Here's how the part is built. I have some questions about the finished solid (model axes, mm). A direction names the side the tool comes from. Coordinates: 2 decimals unless noted, no trailing zeros. Write each loop counter-clockwise with the first axis right and the second up, starting at its lowest first coordinate (ties: lowest second). Pieces come first, ordered by that corner, then holes.
Item 1: Please list where these lines run through material, in increasing order: line 1 (Z direction, x = 13, y = 0); line 2 (Y direction, x = 5.5, z = 0); line 3 (X direction, y = 2.25, z = 13.5).
Item 2: I want a section at C-C (x = 12.5). Please give me the cut outline in (y, z).
Item 3: I'm going to push flat-ended pins straight in: P1, Ø2.5, axis at y = -0.5, z = -12, coming from the +X side; P2, Ø5, axis at x = 5, y = -3.5, coming from the -Z side; P3, Ø1.8, axis at x = 7.5, y = 5, coming from the -Z side; P4, Ø1.5, axis at y = 1, z = 13, coming from the -X side. Where does each tip first touch, or does it pass through?
Item 4: If we mould it in two halves opening along Z, with no side actions, what happens to faces 4 (the face through (8, 6.78, 0)), 5 (the face through (0, 0.1, -5.5)), 6 (the face through (8, 6, 2)), 7 (the face through (14, 0, 15))? For each: pulls with the +Z half, pulls with the -Z half, needs draft (parallel to the pull), parting line crosses it, or undercut.
Item 5: I want a section at A-A (y = 0). Please give me the cut outline in (x, z), and give its area (3 significant figures).
Item 6: I want a section at D-D (x = 7.75). Please give me the cut outline in (y, z), and give its area (3 significant figures).
Item 7: I want a section at B-B (z = 0). Please give me the cut outline in (x, y).
Item 8: For faces 1 (the face through (14, 2.5, 12)), 2 (the face through (2, -2.5, -12)), 3 (the face through (14, -2.5, 12)), which set-ups out of +Z, -Z, +X, -X, +Y, -Y let a thin tool reach every point of the face, with its end or its side?
from build123d import *

# Parameters (mm, degrees)
SKETCH1_R           = 9
BOSS_EXTRUDE1_DEPTH = 17
SKETCH3_W           = 5
SKETCH3_H           = 15
BOSS_EXTRUDE3_DEPTH = 2.5
SKETCH4_R           = 5
CUT_EXTRUDE1_DEPTH  = 25.392621835


with BuildPart() as part:
    # Sketch1 → Boss-Extrude1 (new body)
    with BuildSketch(Plane(origin=(0, 0, 0), x_dir=(0, 0, -1), z_dir=(1, 0, 0))):
        Circle(SKETCH1_R)
        with BuildLine():
            ThreePointArc((5, 0), (-2.738612788, -4.183300133), (-2, 4.582575695))
            Line((-2, 4.582575695), (-2, 6.78))
            Line((-2, 6.78), (2, 6.78))
            Line((2, 6.78), (2, 4.582575695))
            ThreePointArc((2, 4.582575695), (4.183300133, 2.738612788), (5, 0))
        make_face(mode=Mode.SUBTRACT)
    extrude(amount=BOSS_EXTRUDE1_DEPTH)

    # Sketch3 → Boss-Extrude3 (add)
    with BuildSketch(Plane(origin=(0, 0, 0), x_dir=(1, 0, 0), z_dir=(0, 1, 0))):
        with Locations((2.5, 7.5)):
            Rectangle(SKETCH3_W, SKETCH3_H)
        with Locations((14.5, -7.5)):
            Rectangle(SKETCH3_W, SKETCH3_H)
    boss_extrude3 = extrude(amount=BOSS_EXTRUDE3_DEPTH)

    # Mirror1: Boss-Extrude3 across plane
    add(boss_extrude3.mirror(Plane(origin=(0, 0, 0), x_dir=(0, 0, 1), z_dir=(0, -1, 0))))

    # Sketch4 → Cut-Extrude1 (cut, through all)
    with BuildSketch(Plane.ZY):
        Circle(SKETCH4_R)
    extrude(amount=-CUT_EXTRUDE1_DEPTH, mode=Mode.SUBTRACT)


solid = part.part
Answer:
1. line 1: z = -9 to -5, 5 to 15
1. line 2: y = -9 to -5, 6.78 to 9
1. line 3: x = 12 to 17
2. outline: (-2.5, 8.65) arc R9 ccw (long way) to (2.5, 8.65) - (2.5, 15) - (-2.5, 15) - close; hole (4.58, -2) - (6.78, -2) - (6.78, 2) - (4.58, 2) arc R5 ccw (long way) to start
3. P1: stops at x = 5
3. P2: stops at z = -15
3. P3: stops at z = -8.01
3. P4: stops at x = 12
4. face 4: undercut
4. face 5: needs draft
4. face 6: undercut
4. face 7: pulls with the +Z half
5. outline: (0, -15) - (5, -15) - (5, -9) - (17, -9) - (17, -5) - (0, -5) - close; (0, 5) - (17, 5) - (17, 15) - (12, 15) - (12, 9) - (0, 9) - close
5. area: 196 mm2
6. outline: circle Ø18 at (0, 0); hole (4.58, -2) - (6.78, -2) - (6.78, 2) - (4.58, 2) arc R5 ccw (long way) to start
6. area: 168 mm2
7. outline: (0, -9) - (17, -9) - (17, -5) - (0, -5) - close; (0, 6.78) - (17, 6.78) - (17, 9) - (0, 9) - close
8. face 1: +Z, +X, -X, +Y
8. face 2: -Z, +X, -X, -Y
8. face 3: +Z, +X, -X, -Y
